Could you check a few things on this model? Use its own coordinates, in mm. A direction names the side the tool comes from. Coordinates: 2 decimals unless noted, no trailing zeros. Loops run counter-clockwise (first coordinate to the right, second up) from the corner with the lowest first, then second, coordinate; pieces in that order, holes last.
from build123d import *

# Parameters (mm, degrees)
F0_R     = 1.5
F1_DEPTH = 2.8
F2_R     = 2.5
F2_R_2   = 1.5
F3_DEPTH = 2
F4_R     = 1.25
F5_DEPTH = 5


with BuildPart() as f1:
    # F0 (on Top) → F1 (new body)
    with BuildSketch(Plane.XY):
        Circle(F0_R)
    extrude(amount=F1_DEPTH)

    # F2 (on face) → F3 (join)
    with BuildSketch(Plane(origin=(0, 0, 0), x_dir=(1, 0, 0), z_dir=(0, 0, -1))):
        Circle(F2_R)
        Circle(F2_R_2, mode=Mode.SUBTRACT)
        Circle(F2_R_2)
    extrude(amount=F3_DEPTH)

    # F4 (on face) → F5 (join)
    with BuildSketch(Plane(origin=(0, 0, -2), x_dir=(1, 0, 0), z_dir=(0, 0, -1))):
        Circle(F4_R)
    extrude(amount=F5_DEPTH)


solid = f1.part
(1) Which directions (+Z, -Z, +X, -X, +Y, -Y) give clear straight access to the entire face, cutting with the end or side of a thin tool? Please do faces 1 (the face through (0, 0, 2.8)), 2 (the face through (-1, 1, -2)), 3 (the face through (-1.5, 0.07, 1.38)).
Answers:
face 1: +Z, +X, -X, +Y, -Y
face 2: -Z
face 3: +Z
(2) Imagine slicing it at D-D, the plane z = -1. Write out the boundary of the cut face in (x, y).
Answers:
outline: circle Ø5 at (0, 0)
(3) I need wall thicknesses on probe 1 along Y at (x, z) = (-0.05, 1); probe 2 along X at (y, z) = (0, -6). Which ranges of each line are inside material? Lowest first, please.
Answers:
probe 1: y = -1.5 to 1.5
probe 2: x = -1.25 to 1.25
(4) For pin 1 (2 mm diameter, centred on x = 2, z = -2.5, fed in from -Y), with a flat end and sliding along its axis, tell me the tip position at first contact or that it passes through.
Answers:
pin 1: stops at y = -2.23
(5) Imagine slicing it at C-C, the plane z = 2. Write out the boundary of the cut face in (x, y).
Answers:
outline: circle Ø3 at (0, 0)
(6) Imagine slicing it at A-A, the plane y = 0. Write out the boundary of the cut face in (x, z).
Answers:
outline: (-2.5, -2) - (-1.25, -2) - (-1.25, -7) - (1.25, -7) - (1.25, -2) - (2.5, -2) - (2.5, 0) - (1.5, 0) - (1.5, 2.8) - (-1.5, 2.8) - (-1.5, 0) - (-2.5, 0) - close
